Part model, mm, in its own coordinate system. A direction names the side the tool comes from. Round coordinates to 2 decimals unless told otherwise and drop trailing zeros. Order: outer loops, then holes, each group sorted by start corner. A loop starts at its lowest first (then second) coordinate and runs counter-clockwise, first axis right, second up. Notation, with made-up numbers: (87, 42) -> (103, 42) arc R5 cw to (103, 47) -> close; hole circle Ø9 at (61, -18.5). An arc over 180 degrees is marked (long way). Use CSV: the item, a comma, the result in double quotes.
```python
from build123d import *

# Parameters (mm, degrees)
BOSS_EXTRUDE1_DEPTH         = 152.4
BOSS_EXTRUDE1_DEPTH_BACK    = 152.4
F_1_4_0_25_DIAMETER_HOLE1_D = 6.35


with BuildPart() as part:
    # Sketch4 → Boss-Extrude1 (new, two sides: drawn at the far end of the back side and taken through both)
    with BuildSketch(Plane.XY.offset(-BOSS_EXTRUDE1_DEPTH_BACK)):
        with BuildLine():
            Line((6.35, -5.715), (6.35, 5.715))
            ThreePointArc((6.35, 5.715), (6.164012806, 6.164012806), (5.715, 6.35))
            Line((5.715, 6.35), (-5.715, 6.35))
            ThreePointArc((-5.715, 6.35), (-6.164012806, 6.164012806), (-6.35, 5.715))
            Line((-6.35, 5.715), (-6.35, -5.715))
            ThreePointArc((-6.35, -5.715), (-6.164012806, -6.164012806), (-5.715, -6.35))
            Line((-5.715, -6.35), (5.715, -6.35))
            ThreePointArc((5.715, -6.35), (6.164012806, -6.164012806), (6.35, -5.715))
        make_face()
        with BuildLine():
            Line((4.699, 4.2291), (4.699, -4.2291))
            ThreePointArc((4.699, -4.2291), (4.561369476, -4.561369476), (4.2291, -4.699))
            Line((4.2291, -4.699), (-4.2291, -4.699))
            ThreePointArc((-4.2291, -4.699), (-4.561369476, -4.561369476), (-4.699, -4.2291))
            Line((-4.699, -4.2291), (-4.699, 4.2291))
            ThreePointArc((-4.699, 4.2291), (-4.561369476, 4.561369476), (-4.2291, 4.699))
            Line((-4.2291, 4.699), (4.2291, 4.699))
            ThreePointArc((4.2291, 4.699), (4.561369476, 4.561369476), (4.699, 4.2291))
        make_face(mode=Mode.SUBTRACT)
    extrude(amount=BOSS_EXTRUDE1_DEPTH + BOSS_EXTRUDE1_DEPTH_BACK)

    # 1/4 (0.25) Diameter Hole1 (through all)
    with Locations(Plane.ZY.offset(6.35)):
        with Locations((78.867958923, 0), (111.632041077, 0)):
            Hole(F_1_4_0_25_DIAMETER_HOLE1_D / 2)


solid = part.part
```
(1) Cut at B-B, the plane z = -40. Give the cut face in (x, y) (3 decimals).
Reply:
outline,"(-6.35, -5.715) arc R0.635 ccw to (-5.715, -6.35) -> (5.715, -6.35) arc R0.635 ccw to (6.35, -5.715) -> (6.35, 5.715) arc R0.635 ccw to (5.715, 6.35) -> (-5.715, 6.35) arc R0.635 ccw to (-6.35, 5.715) -> close; hole (-4.699, -4.229) arc R0.47 ccw to (-4.229, -4.699) -> (4.229, -4.699) arc R0.47 ccw to (4.699, -4.229) -> (4.699, 4.229) arc R0.47 ccw to (4.229, 4.699) -> (-4.229, 4.699) arc R0.47 ccw to (-4.699, 4.229) -> close"
(2) Pull direction Y, two halves, no side cores. Call faces 3 (the face through (0, 6.35, -2)), 4 (the face through (-4.699, 0, -2)), 5 (the face through (6.35, 0, -2)): released by +Y, released by -Y, zero draft, split by the parting line, or undercut.
Reply:
face 3,"released by +Y"
face 4,"undercut"
face 5,"zero draft"
(3) Which spindle directions (+Z, -Z, +X, -X, +Y, -Y) get a long thin tool onto all of the face, cutting with end or side? Do faces 1 (the face through (0, -4.699, -2)), 2 (the face through (0, -6.35, -2)). Say none if no direction does.
Reply:
face 1,"+Z, -Z"
face 2,"+Z, -Z, +X, -X, -Y"
(4) Cut at A-A, the plane x = 0.75. Give the cut face in (y, z).
Reply:
outline,"(-6.35, -152.4) -> (-4.7, -152.4) -> (-4.7, 152.4) -> (-6.35, 152.4) -> close; (4.7, -152.4) -> (6.35, -152.4) -> (6.35, 152.4) -> (4.7, 152.4) -> close"
(5) Drop a flat-ended pin along its axis: P1, Ø5, axis at y = 0, z = 78.87, coming from the +X side. Give the stop position or say it passes through.
Reply:
P1,"through"
(6) Probe probe 1 along Y at (x, z) = (-2, 54); probe 2 along Y at (x, z) = (4.5, 40.5). List the from-to ranges inside material, lowest first. Write a range as [from, to].
Reply:
probe 1,"[-6.35, -4.7], [4.7, 6.35]"
probe 2,"[-6.35, -4.61], [4.61, 6.35]"
(7) Cut at C-C, the plane y = 0. Give the cut face in (x, z).
Reply:
outline,"(-6.35, -152.4) -> (-4.7, -152.4) -> (-4.7, 75.69) -> (-6.35, 75.69) -> close; (-6.35, 82.04) -> (-4.7, 82.04) -> (-4.7, 108.46) -> (-6.35, 108.46) -> close; (-6.35, 114.81) -> (-4.7, 114.81) -> (-4.7, 152.4) -> (-6.35, 152.4) -> close; (4.7, -152.4) -> (6.35, -152.4) -> (6.35, 75.69) -> (4.7, 75.69) -> close; (4.7, 82.04) -> (6.35, 82.04) -> (6.35, 108.46) -> (4.7, 108.46) -> close; (4.7, 114.81) -> (6.35, 114.81) -> (6.35, 152.4) -> (4.7, 152.4) -> close"
